Could you check a few things on this model? Use its own coordinates, in mm. Round coordinates to 2 decimals unless told otherwise and drop trailing zeros. Loops run counter-clockwise (first coordinate to the right, second up) from the corner with the lowest first, then second, coordinate; pieces in that order, holes last. Notation, with made-up numbers: (39.5, -16.5) -> (77.5, -16.5) arc R36 cw to (77.5, 21.5) -> close; hole circle Ø1 at (84.5, 28). An arc over 180 degrees is marked (long way). One line per item, written item: value.
```python
from build123d import *

# Parameters (mm, degrees)
BOSS_EXTRUDE1_DEPTH = 3.175
SKETCH2_R           = 6.35
CUT_EXTRUDE1_DEPTH  = 118.131253835
CHAMFER1_SIZE       = 4.399409051
CHAMFER1_SIZE_2     = 2.54


with BuildPart() as part:
    # Sketch1 → Boss-Extrude1 (new body)
    with BuildSketch(Plane.XY):
        Polygon((-57.15, 25.4), (57.15, 25.4), (114.3, 20.6375), (114.3, -20.6375), (57.15, -25.4), (-57.15, -25.4), (-114.3, -20.6375), (-114.3, 20.6375), align=None)
    extrude(amount=BOSS_EXTRUDE1_DEPTH)

    # Sketch2 → Cut-Extrude1 (cut, through all)
    with BuildSketch(Plane.XY.offset(3.175)):
        Circle(SKETCH2_R)
    extrude(amount=-CUT_EXTRUDE1_DEPTH, mode=Mode.SUBTRACT)

    # Chamfer1
    # the kernel refuses this chamfer: 4.399409051, 2.54 mm, written as the material it takes off along each edge
    with BuildSketch(Plane(origin=(23.12299944, 28.23558338, 0), x_dir=(0, 0, 1), z_dir=(0.9965457582448797, -0.0830454798537405, 0))) as chamfer1_piece_1:
        Polygon((CHAMFER1_SIZE, 0), (0, CHAMFER1_SIZE_2), (0, 0), align=None)
    extrude(amount=102.874688123, mode=Mode.SUBTRACT)
    with BuildSketch(Plane(origin=(-23.12299944, -28.23558338, 0), x_dir=(0.0830454798537407, 0.9965457582448796, 0), z_dir=(-0.9965457582448797, 0.08304547985374071, 0))) as chamfer1_piece_2:
        Polygon((CHAMFER1_SIZE_2, 0), (0, -CHAMFER1_SIZE), (0, 0), align=None)
    extrude(amount=102.874688123, mode=Mode.SUBTRACT)
    with BuildSketch(Plane(origin=(-125.64233352, 19.69230554, 3.175), x_dir=(0, 0, -1), z_dir=(0.9965457582448797, 0.08304547985374024, 0))) as chamfer1_piece_3:
        Polygon((CHAMFER1_SIZE_2, 0), (0, -CHAMFER1_SIZE), (0, 0), align=None)
    extrude(amount=125.637985093, mode=Mode.SUBTRACT)
    with BuildSketch(Plane(origin=(125.64233352, -19.69230554, 3.175), x_dir=(-0.08304547985374047, 0.9965457582448795, 0), z_dir=(-0.9965457582448797, -0.0830454798537405, 0))) as chamfer1_piece_4:
        Polygon((CHAMFER1_SIZE, 0), (0, CHAMFER1_SIZE_2), (0, 0), align=None)
    extrude(amount=125.637985093, mode=Mode.SUBTRACT)


solid = part.part
```
Item 1: If we section it at D-D on x = 93: List the corners of the cut face in (y, z) for me (1 decimal), plus the area to 3 significant figures.
Output:
outline: (-22.4, 0) -> (19.9, 0) -> (21.7, 3.2) -> (-18, 3.2) -> (-22.4, 0.6) -> close
area: 132 mm²
Item 2: If we section it at B-B on y = 0: List the corners of the cut face in (x, z) for me (3 decimals).
Output:
outline: (-114.3, 0) -> (-6.35, 0) -> (-6.35, 3.175) -> (-114.3, 3.175) -> close; (6.35, 0) -> (114.3, 0) -> (114.3, 3.175) -> (6.35, 3.175) -> close
Item 3: If we section it at A-A on x = 0: List the corners of the cut face in (y, z) for me (3 decimals), plus the area to 3 significant figures.
Output:
outline: (-25.4, 0) -> (-6.35, 0) -> (-6.35, 3.175) -> (-25.4, 3.175) -> close; (6.35, 0) -> (25.4, 0) -> (25.4, 3.175) -> (6.35, 3.175) -> close
area: 121 mm²
Item 4: If we section it at C-C on z = 2.6: List the corners of the cut face in (x, y) for me (3 decimals), plus the area to 3 significant figures.
Output:
outline: (-114.3, -19.595) -> (-44.64, -25.4) -> (16.167, -25.4) -> (114.3, -17.222) -> (114.3, 19.595) -> (44.64, 25.4) -> (-16.167, 25.4) -> (-114.3, 17.222) -> close; hole circle Ø12.7 at (0, 0)
area: 10,300 mm²
Item 5: If we mould it in two halves opening along X, with no side actions, what happens to faces 1 (the face through (-79.641, -21.884, 1.565)), 2 (the face through (2, -11, 3.175)), 3 (the face through (79.64, 21.91, 1.61)), 4 (the face through (-1.38, -6.2, 1.61))? For each: released by +X, released by -X, zero draft, split by the parting line, or undercut.
Output:
face 1: released by -X
face 2: zero draft
face 3: released by +X
face 4: undercut
Item 6: I need wall thicknesses on line 1 (Y direction, x = 0, z = 2.2); line 2 (X direction, y = 5.5, z = 2.25); line 3 (X direction, y = 4.5, z = 2.9). Which ranges of each line are inside material? Lowest first, please. Write a range as from..to.
Output:
line 1: y = -25.4..-6.35, 6.35..25.4
line 2: x = -114.3..-3.17, 3.17..114.3
line 3: x = -114.3..-4.48, 4.48..114.3
